Autodesk Inventor part; units mm, degrees
ref_plane "YZ Plane" through (0, 0, 0) normal (1, 0, 0) x (0, 1, 0)
ref_plane "XZ Plane" through (0, 0, 0) normal (0, 1, 0) x (-1, 0, 0)
ref_plane "XY Plane" through (0, 0, 0) normal (0, 0, 1) x (1, 0, 0)
sketch "Sketch1" plane through (0, 0, 0) normal (0, 1, 0) x (-1, 0, 0)
  line L0 (0, 0) -> (0, -160) construction
  line L1 (5, 0) -> (5, -160)
  line L2 (-5, -160) -> (-5, 0)
  arc A0 (5, 0) -> (-5, 0) centre (0, 0) ccw
  arc A1 (-5, -160) -> (5, -160) centre (0, -160) ccw
  circle A2 centre (0, 0) radius 1.65
  line L3 (0, -30) -> (0, -120) construction
  line L4 (1.65, -30) -> (1.65, -120)
  line L5 (-1.65, -120) -> (-1.65, -30)
  arc A3 (1.65, -30) -> (-1.65, -30) centre (0, -30) ccw
  arc A4 (-1.65, -120) -> (1.65, -120) centre (0, -120) ccw
  point P0 (0, -80)
  point P1 (0, -75)
  dimension "d0" = 160
  dimension "d1" = 10
  dimension "d2" = 3.3
  dimension "d3" = 30
  dimension "d5" = 120
  dimension "d6" = 3.3
extrude "Extrusion1" add sketch "Sketch1" along normal blind 6
sketch "Sketch2" plane through (5, 0, 0) normal (1, 0, 0) x (0, 0, -1)
  line L0 (160, 0) -> (160, 6)
  line L1 (0, 0) -> (160, 0)
  line L2 (160, 0) -> (160, 6)
  line L3 (0, 6) -> (160, 6)
  line L4 (0, 0) -> (0, 6)
  line L5 (160, 0) -> (160, 0)
  line L6 (160, 0) -> (160, 6)
  line L7 (160, 6) -> (160, 6)
  line L8 (160, 0) -> (160, 6)
  line L9 (160, 0) -> (0, 0)
  arc A0 (373.775, -84) -> (160, 0) centre (160, -314.0223) ccw
  line L10 (160, 6) -> (0, 6)
  arc A1 (373.775, -78) -> (160, 6) centre (160, -308.0223) ccw
  line L11 (373.775, -78) -> (373.775, -84)
  line L12 (0, 0) -> (160, 0)
  dimension "d9" = 6
  dimension "d10" = 373.775
  dimension "d11" = 90
extrude "Extrusion2" add sketch "Sketch2" against normal blind 10 contours L0 A1 L11 A0
fillet "Fillet1" radius 2 4 edges at (0, -78, -373.775) (5, -81, -373.775) (-5, -81, -373.775) (0, -84, -373.775)
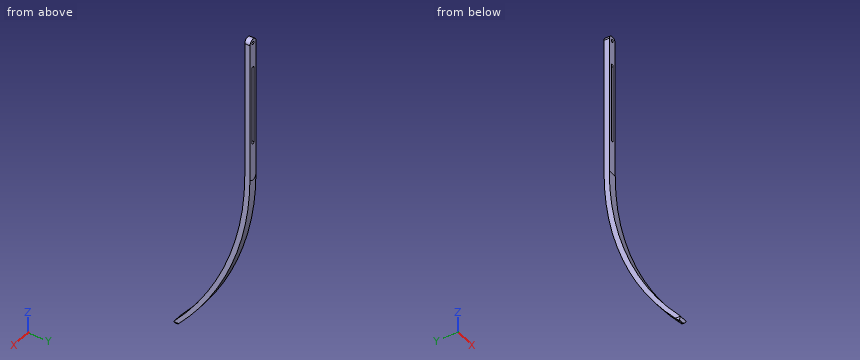
Could you check a few things on this model? Use its own coordinates, in mm. Give positions to 0.01 mm unless a question says otherwise; leave off trailing zeros. Order: outer loops, then holes, each group sorted by start corner. A loop starts at its lowest first (then second) coordinate and runs counter-clockwise, first axis right, second up. Notation, with made-up numbers: (8, 39) - (34, 39) arc R19 cw to (34, 56) - close; hole circle Ø7 at (29.5, -5). An arc over 180 degrees is marked (long way). One line per item, written item: value. Start each with the question number.
1. Imagine slicing it at D-D on z = -231. List the corners of the cut face in (x, y) for me.
2. Imagine slicing it at B-B on x = 0. Give the number of separate pieces and of enclosed holes in the cut face, plus the area to 3 significant figures.
3. If I drill on probe 1 along Y at (x, z) = (-3.75, -94); probe 2 along Z at (x, y) = (-4.25, -55); probe 3 along Z at (x, y) = (2.5, -45), over which ranges is the centre line in solid material (lowest first)?
4. Imagine slicing it at C-C on y = -25.5. List the corners of the cut face in (x, z) for me, plus the area to 3 significant figures.
5. For P1, Ø1.5, axis at x = -3.5, y = -47.5, coming from the -Z side; P2, Ø2, axis at x = 1.5, z = -59.5, coming from the +Y side; P3, Ø4, axis at x = 0, z = 0, coming from the -Y side; P4, Ø4, axis at x = 1, z = -272.5, coming from the +Y side, each with a flat end and sliding along its axis, tell me the tip position at first contact or that it passes through.
6. Imagine slicing it at A-A on z = -41. List the corners of the cut face in (x, y) for me.
Values:
1. outline: (-5, -8.13) - (5, -8.13) - (5, -2.13) - (-5, -2.13) - close
2. separate pieces: 3
2. enclosed holes: 0
2. area: 1,690 mm²
3. probe 1: 0 to 6
3. probe 2: -345.98 to -337.53
3. probe 3: -331.55 to -321.98
4. outline: (-5, -297.08) - (5, -297.08) - (5, -283.96) - (-5, -283.96) - close
4. area: 131 mm²
5. P1: z = -336.43
5. P2: y = 6
5. P3: y = 0
5. P4: y = -14.08
6. outline: (-5, 0) - (-1.65, 0) - (-1.65, 6) - (-5, 6) - close; (1.65, 0) - (5, 0) - (5, 6) - (1.65, 6) - close
